```python
from build123d import *

# Parameters (mm, degrees)
SKETCH_1_R      = 1.5
SKETCH_1_R_2    = 1.55
SKETCH_1_R_3    = 8
SKETCH_1_R_4    = 1.555
SKETCH_1_R_5    = 3
SKETCH_1_R_6    = 17.486246266
SKETCH_1_R_7    = 17.020495335
SKETCH_1_R_8    = 16.467245603
SKETCH_1_R_9    = 13.84365186
SKETCH_1_R_10   = 12.763304461
SKETCH_1_R_11   = 13.972809186
SKETCH_1_R_12   = 7.02721673
SKETCH_1_R_13   = 8.054225091
SKETCH_1_R_14   = 7.029505311
SKETCH_1_R_15   = 5.06480667
SKETCH_1_R_16   = 5.84755638
SKETCH_1_R_17   = 4.172193425
SKETCH_1_R_18   = 7.080536247
SKETCH_1_R_19   = 7.569466987
SKETCH_1_R_20   = 6.673296635
SKETCH_1_R_21   = 7.63323109
SKETCH_1_R_22   = 6.378997066
SKETCH_1_R_23   = 6.842517181
SKETCH_1_R_24   = 5.589183479
SKETCH_1_W      = 30
SKETCH_1_H      = 6.05
SKETCH_1_H_2    = 6.25
EXTRUDE_1_DEPTH = 1.5


with BuildPart() as part:
    # 草图1 → 凸台-拉伸1 (new body)
    with BuildSketch(Plane(origin=(0, 0, 0), x_dir=(1, 0, 0), z_dir=(0, 1, 0))):
        Polygon((0, -33), (82.892637189, -84.836900302), (139.996166095, -84.836900302), (219.992332189, -33), (219.992332189, 0), (139.996166095, 53.713791291), (82.892637189, 53.713791291), (0, 0), align=None)
        with Locations((6, -27.75)):
            Circle(SKETCH_1_R, mode=Mode.SUBTRACT)
        with Locations((6, -5.45)):
            Circle(SKETCH_1_R, mode=Mode.SUBTRACT)
        with Locations((24.5, -8.7)):
            Circle(SKETCH_1_R, mode=Mode.SUBTRACT)
        with Locations((24.5, -24.3)):
            Circle(SKETCH_1_R, mode=Mode.SUBTRACT)
        with Locations((195.5, -8.7)):
            Circle(SKETCH_1_R, mode=Mode.SUBTRACT)
        with Locations((195.5, -24.3)):
            Circle(SKETCH_1_R, mode=Mode.SUBTRACT)
        with Locations((214, -27.75)):
            Circle(SKETCH_1_R, mode=Mode.SUBTRACT)
        with Locations((214, -5.45)):
            Circle(SKETCH_1_R, mode=Mode.SUBTRACT)
        with Locations((105.046418626, -21.449747468)):
            Circle(SKETCH_1_R_2, mode=Mode.SUBTRACT)
        with Locations((114.945913563, -21.449747468)):
            Circle(SKETCH_1_R_2, mode=Mode.SUBTRACT)
        with Locations((10, -16.5)):
            Circle(SKETCH_1_R_3, mode=Mode.SUBTRACT)
        with Locations((210, -16.5)):
            Circle(SKETCH_1_R_3, mode=Mode.SUBTRACT)
        with Locations((114.742384657, -11.753781438)):
            Circle(SKETCH_1_R_2, mode=Mode.SUBTRACT)
        with Locations((83.096166095, 38.5)):
            Circle(SKETCH_1_R_2, mode=Mode.SUBTRACT)
        with Locations((105.046418626, -11.550252532)):
            Circle(SKETCH_1_R_2, mode=Mode.SUBTRACT)
        with Locations((102.996166095, -16.5)):
            Circle(SKETCH_1_R_2, mode=Mode.SUBTRACT)
        with Locations((109.996166095, -23.5)):
            Circle(SKETCH_1_R_4, mode=Mode.SUBTRACT)
        with Locations((116.996166095, -16.5)):
            Circle(SKETCH_1_R_2, mode=Mode.SUBTRACT)
        with Locations((109.996166095, -9.5)):
            Circle(SKETCH_1_R_2, mode=Mode.SUBTRACT)
        with Locations((109.996166095, -16.5)):
            Circle(SKETCH_1_R_5, mode=Mode.SUBTRACT)
        with Locations((129.195913563, -21.449747468)):
            Circle(SKETCH_1_R_2, mode=Mode.SUBTRACT)
        with Locations((128.992384657, -11.753781438)):
            Circle(SKETCH_1_R_2, mode=Mode.SUBTRACT)
        with Locations((137.896166095, 38.5)):
            Circle(SKETCH_1_R_2, mode=Mode.SUBTRACT)
        with Locations((137.896166095, -71.5)):
            Circle(SKETCH_1_R_2, mode=Mode.SUBTRACT)
        with Locations((83.096166095, -71.5)):
            Circle(SKETCH_1_R_2, mode=Mode.SUBTRACT)
        with Locations((105.046418626, 18.503675588)):
            Circle(SKETCH_1_R_6, mode=Mode.SUBTRACT)
        with Locations((105.046418626, -52.199044439)):
            Circle(SKETCH_1_R_7, mode=Mode.SUBTRACT)
        with Locations((150.29958532, -48.585783177)):
            Circle(SKETCH_1_R_8, mode=Mode.SUBTRACT)
        with Locations((55.978889615, 14.234912262)):
            Circle(SKETCH_1_R_9, mode=Mode.SUBTRACT)
        with Locations((161.159046839, 16.460208899)):
            Circle(SKETCH_1_R_10, mode=Mode.SUBTRACT)
        with Locations((54.344707062, -48.585783177)):
            Circle(SKETCH_1_R_11, mode=Mode.SUBTRACT)
        with Locations((116.996166095, 41.77756602)):
            Circle(SKETCH_1_R_12, mode=Mode.SUBTRACT)
        with Locations((75.041941004, -15.050367065)):
            Circle(SKETCH_1_R_13, mode=Mode.SUBTRACT)
        with Locations((85.237439413, -29.806396783)):
            Circle(SKETCH_1_R_14, mode=Mode.SUBTRACT)
        with Locations((87.36558551, -1.911662428)):
            Circle(SKETCH_1_R_15, mode=Mode.SUBTRACT)
        with Locations((128.992384657, -1.911662428)):
            Circle(SKETCH_1_R_16, mode=Mode.SUBTRACT)
        with Locations((145.020577925, -1.911662428)):
            Circle(SKETCH_1_R_17, mode=Mode.SUBTRACT)
        with Locations((185, 3.935893952)):
            Circle(SKETCH_1_R_18, mode=Mode.SUBTRACT)
        with Locations((177.919463753, -41.321628131)):
            Circle(SKETCH_1_R_19, mode=Mode.SUBTRACT)
        with Locations((26.38546357, 3.153144243)):
            Circle(SKETCH_1_R_20, mode=Mode.SUBTRACT)
        with Locations((24.5, -36.835902094)):
            Circle(SKETCH_1_R_21, mode=Mode.SUBTRACT)
        with Locations((75.041941004, -52.199044439)):
            Circle(SKETCH_1_R_22, mode=Mode.SUBTRACT)
        with Locations((121.206538505, -76.107131723)):
            Circle(SKETCH_1_R_23, mode=Mode.SUBTRACT)
        with Locations((123.144828277, -33)):
            Circle(SKETCH_1_R_24, mode=Mode.SUBTRACT)
        with Locations((170, -8.475)):
            Rectangle(SKETCH_1_W, SKETCH_1_H, mode=Mode.SUBTRACT)
        with Locations((170, -24.625)):
            Rectangle(SKETCH_1_W, SKETCH_1_H_2, mode=Mode.SUBTRACT)
        with Locations((50, -24.625)):
            Rectangle(SKETCH_1_W, SKETCH_1_H_2, mode=Mode.SUBTRACT)
        with Locations((50, -8.475)):
            Rectangle(SKETCH_1_W, SKETCH_1_H, mode=Mode.SUBTRACT)
    extrude(amount=EXTRUDE_1_DEPTH)


solid = part.part
```
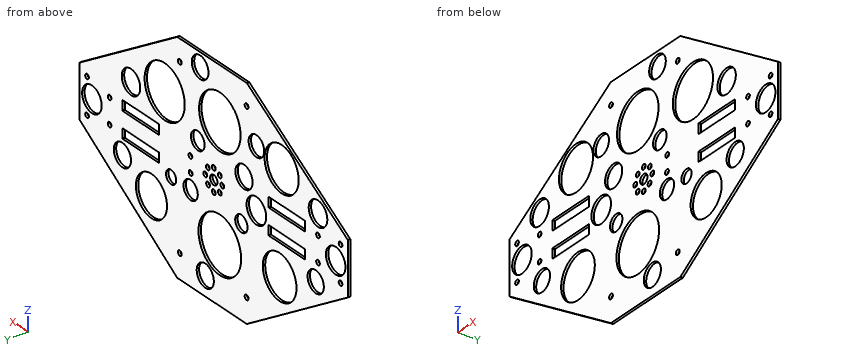
Part model, mm, in its own coordinate system. Give positions to 0.01 mm unless a question says otherwise; leave off trailing zeros. Use one line per item in the form item = value.
Item 1: Pin check, flat tips, straight feed: pin 1 Ø13 at (x, z) = (123.14, 33) entering from +Y; pin 2 Ø14.5 at (x, z) = (10, 16.5) entering from -Y; pin 3 Ø0.8 at (x, y) = (173.5, 1) entering from -Z. Stop position of each tip, or through.
Solution:
pin_1 = 1.5
pin_2 = through
pin_3 = -31.49
Item 2: Probe probe 1 along Z at (x, y) = (80.5, 0.8); probe 2 along X at (y, z) = (0.5, -8); probe 3 along X at (y, z) = (0.3, -10). List the from-to ranges inside material, lowest first. Write a range as from..to.
Solution:
probe_1 = -52.16..9.13, 20.97..24.61, 35..48.9, 55.5..83.34
probe_2 = 12.35..21.8, 30.97..43.62, 68.34..91.07, 119.03..151.6, 170.72..179.2, 190.8..208.08
probe_3 = 15.43..42.8, 69.16..89.77, 120.33..150.15, 172.17..181.34, 188.66..205.1
Item 3: Slice it at A-A on y = 0.4. Count the separate pieces of the cut face and the enclosed holes in it, and give its area (3 significant figures).
Solution:
separate_pieces = 1
enclosed_holes = 48
area = 14,300 mm2
